Verification items for the finished model (mm, model axes). A direction names the side the tool comes from. Give positions to 0.01 mm unless a question says otherwise; leave off trailing zeros. Order: outer loops, then holes, each group sorted by start corner. A loop starts at its lowest first (then second) coordinate and runs counter-clockwise, first axis right, second up.
(1) Sectioned sample at D-D on y = 52.5. Record the cut outline in (x, z) (3 decimals), plus the area to 3 significant figures.
(2) Scan lines: L1, parallel to Z at x = -5, y = -19 (3 decimals); L2, parallel to Y at x = 4, z = 51 (3 decimals); L3, parallel to X at y = 6.5, z = -2 (3 decimals). Record each from-to range of solid material in increasing order.
(3) Sectioned sample at A-A on y = 14. Record the cut outline in (x, z) (3 decimals), plus the area to 3 significant figures.
(4) Gauge pin test, flat ends, axial feed: pin 1 (5 mm diameter, centred on x = 24.5, y = -5, fed in from +Z); pin 2 (22 mm diameter, centred on x = 76, y = 11.5, fed in from -Z); pin 3 (12 mm diameter, centred on y = 15, z = 31, fed in from -X) (3 decimals). Record the tip position at first contact, or that the pin passes through.
(5) Sectioned sample at B-B on x = 61. Record the cut outline in (y, z), plus the area to 3 significant figures.
(6) Sectioned sample at C-C on z = 1. Record the cut outline in (x, y) (3 decimals).
(7) Access from +Z, -Z, +X, -X, +Y, -Y to the whole of each face (thin tool, end or side, straight path). Record for faces 1 (the face through (22.225, -14, 26)), 2 (the face through (39.37, 41.5, 7.71)), 3 (the face through (32.73, 13.58, 66.37)).
```python
from build123d import *

# Parameters (mm, degrees)
F1_DEPTH = 63.5
F0_W     = 25.4
F0_H     = 9.398
F2_DEPTH = 25.4
F3_DEPTH = 8.255
F4_R     = 6.35
F5_R     = 6.35


with BuildPart() as f1:
    # F0 (on Front) → F1 (new body, symmetric)
    with BuildSketch(Plane.XZ):
        Polygon((22.225, 9.525), (-41.275, 9.525), (-41.275, -9.525), (41.275, -9.525), (41.275, 9.525), align=None)
    extrude(amount=F1_DEPTH, both=True)

    # F0 (on Front) → F2 (join, symmetric)
    with BuildSketch(Plane.XZ):
        with BuildLine():
            Line((22.225, 41.402), (22.225, 9.525))
            Line((22.225, 9.525), (41.275, 9.525))
            Line((41.275, 9.525), (41.275, 41.402))
            ThreePointArc((41.275, 41.402), (45.9246798487, 52.6273201513), (57.15, 57.277))
            Line((57.15, 57.277), (59.0423882883, 57.277))
            Line((59.0423882883, 57.277), (59.0423882883, 66.675))
            Line((59.0423882883, 66.675), (84.4423882883, 66.675))
            Line((84.4423882883, 66.675), (84.4423882883, 76.327))
            Line((84.4423882883, 76.327), (57.15, 76.327))
            ThreePointArc((57.15, 76.327), (32.4542956671, 66.0977043329), (22.225, 41.402))
        make_face()
        with Locations((71.7423882883, 61.976)):
            Rectangle(F0_W, F0_H)
    extrude(amount=F2_DEPTH, both=True)

    # F0 (on Front) → F3 (join, symmetric)
    with BuildSketch(Plane.XZ):
        with BuildLine():
            add(Edge.make_bspline(
                [(-41.275, 9.525), (-40.4969751835, 44.2796610296), (12.460607104, 76.7662450671), (57.15, 76.327)],
                knots=[0, 0, 0, 0, 118.9537213752, 118.9537213752, 118.9537213752, 118.9537213752], degree=3))
            Line((-41.275, 9.525), (22.225, 9.525))
            Line((22.225, 9.525), (22.225, 41.402))
            ThreePointArc((22.225, 41.402), (32.4542956671, 66.0977043329), (57.15, 76.327))
        make_face()
    extrude(amount=F3_DEPTH, both=True)

    # F4
    f4_edges = [f1.edges().sort_by_distance(p)[0] for p in [
        (41.275, -44.45, 9.525),
        (41.275, -63.5, 0),
        (41.275, 44.45, 9.525),
        (41.275, 63.5, 0),
        (0, 63.5, 9.525),
        (0, -63.5, 9.525),
        (-41.275, -35.8775, 9.525),
        (-41.275, 35.8775, 9.525),
        (0, -63.5, -9.525),
        (-41.275, -63.5, 0),
        (-41.275, 63.5, 0),
    ]]
    fillet(f4_edges, radius=F4_R)

    # F5
    f5_edges = [f1.edges().sort_by_distance(p)[0] for p in [
        (84.442388, -25.4, 66.802),
        (70.796194, -25.4, 76.327),
        (84.442388, 0, 76.327),
        (70.796194, 25.4, 76.327),
    ]]
    fillet(f5_edges, radius=F5_R)


solid = f1.part
```
Ans:
1. outline: (-41.275, -9.525) - (41.275, -9.525) - (41.275, 3.175) arc R6.35 ccw to (34.925, 9.525) - (-34.925, 9.525) arc R6.35 ccw to (-41.275, 3.175) - close
1. area: 1,560 mm2
2. L1: z = -9.525 to 9.525
2. L2: y = -8.255 to 8.255
2. L3: x = -41.275 to 41.275
3. outline: (-41.275, -9.525) - (41.275, -9.525) - (41.275, 41.402) arc R15.875 cw to (57.15, 57.277) - (84.442, 57.277) - (84.442, 69.977) arc R6.35 ccw to (78.092, 76.327) - (57.15, 76.327) arc R34.925 ccw to (22.225, 41.402) - (22.225, 9.525) - (-34.925, 9.525) arc R6.35 ccw to (-41.275, 3.175) - close
3. area: 3,440 mm2
4. pin 1: stops at z = 72.14
4. pin 2: stops at z = 57.28
4. pin 3: stops at x = 22.225
5. outline: (-25.4, 57.28) - (25.4, 57.28) - (25.4, 69.98) arc R6.35 ccw to (19.05, 76.33) - (-19.05, 76.33) arc R6.35 ccw to (-25.4, 69.98) - close
5. area: 950 mm2
6. outline: (-41.275, -57.15) arc R6.35 ccw to (-34.925, -63.5) - (34.925, -63.5) arc R6.35 ccw to (41.275, -57.15) - (41.275, 57.15) arc R6.35 ccw to (34.925, 63.5) - (-34.925, 63.5) arc R6.35 ccw to (-41.275, 57.15) - close
7. face 1: +Z, -X, -Y
7. face 2: +Z, +X, +Y
7. face 3: +Z, -X, +Y
